```python
from build123d import *

# Parameters (mm, degrees)
F1_DEPTH = 25
F2_W     = 20
F2_H     = 20
F3_DEPTH = 10
F3_TAPER = 5
F5_DEPTH = 5
F6_R     = 4
F6_R_2   = 2.5
F7_DEPTH = 6
F8_DEPTH = 45
F9_R     = 1
F10_R    = 3


with BuildPart() as f1:
    # F0 (on Front) → F1 (new body, symmetric)
    with BuildSketch(Plane.XZ):
        Polygon((-50, 25), (-50, 0), (50, 0), (50, 25), (20, 42.3205080757), (-20, 42.3205080757), align=None)
    extrude(amount=F1_DEPTH, both=True)

    # F2 (on face) → F3 (join)
    with BuildSketch(Plane.XY.offset(42.3205080757)):
        Rectangle(F2_W, F2_H)
    extrude(amount=F3_DEPTH, taper=F3_TAPER)

    # F4 (on face) → F5 (join)
    with BuildSketch(Plane.XY.offset(52.3205080757)):
        Polygon((-6.2786841774, -3.625), (0, -7.25), (6.2786841774, -3.625), (6.2786841774, 3.625), (0, 7.25), (-6.2786841774, 3.625), align=None)
    extrude(amount=F5_DEPTH)

    # F6 (on face) → F7 (join)
    with BuildSketch(Plane.XY.offset(57.3205080757)):
        with Locations((-0.0816522495, -0.0350918563)):
            Circle(F6_R)
        with Locations((-0.0816522495, -0.0350918563)):
            Circle(F6_R_2, mode=Mode.SUBTRACT)
    extrude(amount=F7_DEPTH)

    # F8 (cut): a face of the model
    f8_faces = [f1.faces().sort_by_distance(p)[0] for p in [
        (-0.0816522495, -0.0350918563, 57.3205080757),
    ]]
    extrude(f8_faces, amount=-F8_DEPTH, mode=Mode.SUBTRACT)

    # F9
    f9_edges = [f1.edges().sort_by_distance(p)[0] for p in [
        (0, -9.125113, 52.320508),
        (-9.125113, 0, 52.320508),
        (9.125113, 0, 52.320508),
        (0, 9.125113, 52.320508),
        (-4.081652, -0.035092, 57.320508),
    ]]
    fillet(f9_edges, radius=F9_R)

    # F10
    f10_edges = [f1.edges().sort_by_distance(p)[0] for p in [
        (-20, 0, 42.320508),
        (20, 0, 42.320508),
    ]]
    fillet(f10_edges, radius=F10_R)


solid = f1.part
```
CAD build for the part. Positions are in the model's coordinates, mm. A direction names the side the tool comes from. Round coordinates to 2 decimals unless told otherwise and drop trailing zeros. Write each loop counter-clockwise with the first axis right and the second up, starting at its lowest first coordinate (ties: lowest second). Pieces come first, ordered by that corner, then holes. Notation, with made-up numbers: (6.25, 69.25) -> (57.25, 69.25) arc R5 ccw to (57.25, 75.25) -> close; hole circle Ø3 at (44, 0.25). An arc over 180 degrees is marked (long way). Answer in a Markdown table with one row per item. Add a question column.
Item 1: Which spindle directions (+Z, -Z, +X, -X, +Y, -Y) get a long thin tool onto all of the face, cutting with end or side? Do faces 5 (the face through (3.183, 5.412, 54.786)), 6 (the face through (2, -5, 57.321)), 7 (the face through (-3.183, -5.412, 54.786)), 8 (the face through (-6.279, 0, 55)). Say none if no direction does.
Item 2: Saw through at D-D, the plane z = 36. Write the cut outline in (x, y).
Item 3: Saw through at A-A, the plane y = 16.5. Write the cut outline in (x, z).
Item 4: Mould opens along Y. For faces 1 (the face through (0, 0, 12.321)), 2 (the face through (0.14, -9.61, 46.8)), 3 (the face through (-0.624, -2.476, 37.464)), 4 (the face through (-0.95, -3.94, 60.79)) say: pulls with the +Y half, pulls with the -Y half, needs draft (parallel to the pull), parting line crosses it, or undercut.
Item 5: Saw through at C-C, the plane x = -13. Write the cut outline in (y, z), then the cut area to 3 significant figures.
Item 6: Drop flat-ended pins along their axis: pin 1 Ø2 at (y, z) = (16, 41.5) entering from -X; pin 2 Ø1.5 at (x, y) = (27, 11.5) entering from +Z; pin 3 Ø10 at (y, z) = (-17, 47.5) entering from +X; pin 4 Ø4 at (y, z) = (10, 26.5) entering from -X. Give the stop position or say it passes through.
Item 7: Drill centre lines: line 1 (Z direction, x = 11, y = 12.5); line 2 (Z direction, x = -1.5, y = 1.5); line 3 (X direction, y = 8.5, z = 45.5). Where is each one in solid material? Low to high. Write a range as from..to.
Item 8: Saw through at B-B, the plane z = 56. Write the cut outline in (x, y) (3 decimals), then the cut area to 3 significant figures.
Findings below:
| question | item | result |
|---|---|---|
| 1 | face 5 | +Z, +X, +Y |
| 1 | face 6 | +Z |
| 1 | face 7 | +Z, -X, -Y |
| 1 | face 8 | +Z, -X, +Y, -Y |
| 2 | outline | (-30.95, -25) -> (30.95, -25) -> (30.95, 25) -> (-30.95, 25) -> close; hole circle Ø5 at (-0.08, -0.04) |
| 3 | outline | (-50, 0) -> (50, 0) -> (50, 25) -> (20.7, 41.92) arc R3 ccw to (19.2, 42.32) -> (-19.2, 42.32) arc R3 ccw to (-20.7, 41.92) -> (-50, 25) -> close |
| 4 | face 1 | undercut |
| 4 | face 2 | pulls with the -Y half |
| 4 | face 3 | undercut |
| 4 | face 4 | parting line crosses it |
| 5 | outline | (-25, 0) -> (25, 0) -> (25, 42.32) -> (-25, 42.32) -> close |
| 5 | area | 2,120 mm^2 |
| 6 | pin 1 | stops at x = -23.15 |
| 6 | pin 2 | stops at z = 38.71 |
| 6 | pin 3 | passes through |
| 6 | pin 4 | stops at x = -50 |
| 7 | line 1 | z = 0..42.32 |
| 7 | line 2 | z = 0..12.32 |
| 7 | line 3 | x = -9.72..9.72 |
| 8 | outline | (-6.279, -3.625) -> (0, -7.25) -> (6.279, -3.625) -> (6.279, 3.625) -> (0, 7.25) -> (-6.279, 3.625) -> close; hole circle Ø5 at (-0.082, -0.035) |
| 8 | area | 117 mm^2 |
